```python
from build123d import *
from build123d.topology import SkipClean

# Parameters (mm, degrees)
SKETCH1_R           = 75
BOSS_EXTRUDE1_DEPTH = 30
SKETCH2_R           = 30.5
CUT_EXTRUDE1_DEPTH  = 15
BOSS_EXTRUDE2_DEPTH = 105
SKETCH4_R           = 10
CUT_EXTRUDE2_DEPTH  = 105
SKETCH5_R           = 3
CUT_EXTRUDE3_DEPTH  = 105


with BuildPart() as part:
    # Sketch1 → Boss-Extrude1 (new body)
    with BuildSketch(Plane(origin=(0, 0, 0), x_dir=(1, 0, 0), z_dir=(0, 1, 0))):
        with Locations(Location((0, 0, 0), (0, 0, 270))):
            Circle(SKETCH1_R)
    extrude(amount=BOSS_EXTRUDE1_DEPTH)

    # Sketch2 → Cut-Extrude1 (cut)
    with BuildSketch(Plane(origin=(0, 30, 0), x_dir=(1, 0, 0), z_dir=(0, 1, 0))):
        with Locations(Location((0, 0, 0), (0, 0, 270))):
            Circle(SKETCH2_R)
    extrude(amount=-CUT_EXTRUDE1_DEPTH, mode=Mode.SUBTRACT)

    # Sketch3 → Boss-Extrude2 (add)
    with SkipClean():  # the faces are left unmerged after this step: merging them gives an invalid solid
        with BuildSketch(Plane(origin=(0, 30, 0), x_dir=(1, 0, 0), z_dir=(0, 1, 0))):
            with BuildLine():
                Line((43.301270189, 25), (64.951905284, 37.5))
                ThreePointArc((64.951905284, 37.5), (75, 0), (64.951905284, -37.5))
                Line((64.951905284, -37.5), (43.301270189, -25))
                ThreePointArc((43.301270189, -25), (50, 0), (43.301270189, 25))
            make_face()
            with BuildLine():
                Line((-43.301270189, -25), (-64.951905284, -37.5))
                ThreePointArc((-64.951905284, -37.5), (-75, 0), (-64.951905284, 37.5))
                Line((-64.951905284, 37.5), (-43.301270189, 25))
                ThreePointArc((-43.301270189, 25), (-50, 0), (-43.301270189, -25))
            make_face()
        extrude(amount=BOSS_EXTRUDE2_DEPTH)

    # Sketch4 → Cut-Extrude2 (cut)
    with SkipClean():  # the faces are left unmerged after this step: merging them gives an invalid solid
        with BuildSketch(Plane.XZ):
            with Locations(Location((0, 0, 0), (0, 0, 270))):
                Circle(SKETCH4_R)
        extrude(amount=-CUT_EXTRUDE2_DEPTH, mode=Mode.SUBTRACT)

    # Sketch5 → Cut-Extrude3 (cut)
    with SkipClean():  # the faces are left unmerged after this step: merging them gives an invalid solid
        with BuildSketch(Plane.XZ):
            with Locations(Location((-15.733125881, 15.733125881, 0), (0, 0, 270))):
                Circle(SKETCH5_R)
            with Locations(Location((15.733125881, 15.733125881, 0), (0, 0, 270))):
                Circle(SKETCH5_R)
            with Locations(Location((15.733125881, -15.733125881, 0), (0, 0, 270))):
                Circle(SKETCH5_R)
            with Locations(Location((-15.733125881, -15.733125881, 0), (0, 0, 270))):
                Circle(SKETCH5_R)
        extrude(amount=-CUT_EXTRUDE3_DEPTH, mode=Mode.SUBTRACT)


solid = part.part
```
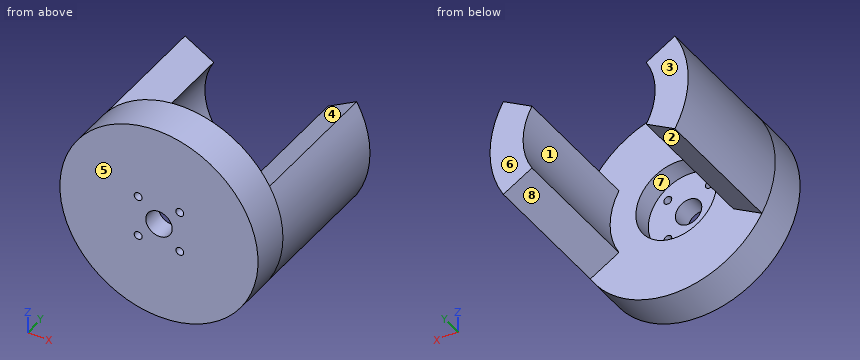
Verification items for the finished model (mm, model axes). Face numbers are marked on the shaded views. A direction names the side the tool comes from. Coordinates: 2 decimals unless noted, no trailing zeros. Write each loop counter-clockwise with the first axis right and the second up, starting at its lowest first coordinate (ties: lowest second). Pieces come first, ordered by that corner, then holes. Notation, with made-up numbers: M 9.5,71 L 18.5,71 A31 cw 18.5,110 Z; hole C -8,66.25 d10. An arc over 180 degrees is marked long. One line per item, written item: value.
Item 1: Scan lines: line 1 along X through (y, z) = (9, 0); line 2 along X through (y, z) = (23, 0); line 3 along Y through (x, z) = (4.5, 32.5). Record each from-to range of solid material in increasing order.
Check sheet entries:
line 1: x = -75 to -10, 10 to 75
line 2: x = -75 to -30.5, 30.5 to 75
line 3: y = 0 to 30
Item 2: Mould release check, pull along Z, two halves, no side actions. Record for the marked faces 1, 2 and 3: pulls with the +Z half, pulls with the -Z half, needs draft (parallel to the pull), parting line crosses it, or undercut.
Check sheet entries:
face 1: undercut
face 2: pulls with the -Z half
face 3: needs draft
Item 3: Section check D-D, the plane z = 52. Record the boundary of the cut face in (x, y).
Check sheet entries:
outline: M -54.05,0 L 54.05,0 L 54.05,30 L -54.05,30 Z
Item 4: Gauge pin test, flat ends, axial feed: pin 1 Ø12 at (y, z) = (97.5, 28.5) entering from -X; pin 2 Ø2 at (x, z) = (-35.5, -20.5) entering from +Y; pin 3 Ø9.5 at (x, z) = (-15.73, -15.73) entering from +Y. Record the tip position at first contact, or that the pin passes through.
Check sheet entries:
pin 1: stops at x = -71.55
pin 2: stops at y = 30
pin 3: stops at y = 15
Item 5: Section check B-B, the plane z = 0. Record the boundary of the cut face in (x, y), plus the area to 4 significant figures.
Check sheet entries:
outline: M -75,0 L -10,0 L -10,15 L -30.5,15 L -30.5,30 L -50,30 L -50,135 L -75,135 Z; M 10,0 L 75,0 L 75,135 L 50,135 L 50,30 L 30.5,30 L 30.5,15 L 10,15 Z
area: 8,535 mm^2
Item 6: Access from +Z, -Z, +X, -X, +Y, -Y to the whole of each face (thin tool, end or side, straight path). Record for the marked faces 4, 5, 6, 7 and 8.
Check sheet entries:
face 4: +Z, +Y
face 5: +Z, -Z, +X, -X, -Y
face 6: +Z, -Z, +X, -X, +Y
face 7: +Y
face 8: -Z, +Y
Item 7: Section check C-C, the plane x = 0. Record the boundary of the cut face in (y, z).
Check sheet entries:
outline: M 0,-75 L 30,-75 L 30,-30.5 L 15,-30.5 L 15,-10 L 0,-10 Z; M 0,10 L 15,10 L 15,30.5 L 30,30.5 L 30,75 L 0,75 Z
Item 8: Section check A-A, the plane y = 53. Record the boundary of the cut face in (x, z), plus the area to 3 significant figures.
Check sheet entries:
outline: M -64.95,-37.5 L -43.3,-25 A50 cw -43.3,25 L -64.95,37.5 A75 ccw Z; M 43.3,-25 L 64.95,-37.5 A75 ccw 64.95,37.5 L 43.3,25 A50 cw Z
area: 3,270 mm^2
